CAD build for the part. Positions are in the model's coordinates, mm. Round coordinates to 2 decimals unless told otherwise and drop trailing zeros. Write each loop counter-clockwise with the first axis right and the second up, starting at its lowest first coordinate (ties: lowest second). Pieces come first, ordered by that corner, then holes. Notation, with made-up numbers: (13.5, -15.5) - (19.5, -15.5) arc R32 ccw to (19.5, 18.5) - close; hole circle Ø11 at (-31.5, 59). An arc over 180 degrees is marked (long way). Answer in a Markdown table with one row per item.
```python
from build123d import *

# Parameters (mm, degrees)
SKETCH_1_R      = 3.2
SKETCH_1_R_2    = 1.6
EXTRUDE_1_DEPTH = 3


with BuildPart() as part:
    # 草图1 → 凸台-拉伸1 (new body)
    with BuildSketch(Plane(origin=(0, 0, 0), x_dir=(1, 0, 0), z_dir=(0, 1, 0))):
        with BuildLine():
            Line((5, 0), (175, 0))
            ThreePointArc((175, 0), (178.535533906, 1.464466094), (180, 5))
            Line((180, 5), (180, 175))
            ThreePointArc((180, 175), (178.535533906, 178.535533906), (175, 180))
            Line((175, 180), (5, 180))
            ThreePointArc((5, 180), (1.464466094, 178.535533906), (0, 175))
            Line((0, 175), (0, 5))
            ThreePointArc((0, 5), (1.464466094, 1.464466094), (5, 0))
        make_face()
        with Locations(Location((8, 172, 0), (0, 0, 270))):
            Circle(SKETCH_1_R, mode=Mode.SUBTRACT)
        with Locations(Location((172, 172, 0), (0, 0, 270))):
            Circle(SKETCH_1_R, mode=Mode.SUBTRACT)
        with Locations(Location((8, 8, 0), (0, 0, 270))):
            Circle(SKETCH_1_R, mode=Mode.SUBTRACT)
        with Locations(Location((172, 8, 0), (0, 0, 270))):
            Circle(SKETCH_1_R, mode=Mode.SUBTRACT)
        with Locations(Location((74.5, 175, 0), (0, 0, 270))):
            Circle(SKETCH_1_R_2, mode=Mode.SUBTRACT)
        with Locations(Location((74.5, 144, 0), (0, 0, 270))):
            Circle(SKETCH_1_R_2, mode=Mode.SUBTRACT)
        with Locations(Location((105.5, 144, 0), (0, 0, 90))):
            Circle(SKETCH_1_R_2, mode=Mode.SUBTRACT)
        with Locations(Location((105.5, 175, 0), (0, 0, 90))):
            Circle(SKETCH_1_R_2, mode=Mode.SUBTRACT)
        with Locations(Location((133.6, 172, 0), (0, 0, 270))):
            Circle(SKETCH_1_R_2, mode=Mode.SUBTRACT)
        with Locations(Location((133.6, 158, 0), (0, 0, 270))):
            Circle(SKETCH_1_R_2, mode=Mode.SUBTRACT)
        with Locations(Location((154, 169.5, 0), (0, 0, 270))):
            Circle(SKETCH_1_R_2, mode=Mode.SUBTRACT)
        with Locations(Location((154, 155.5, 0), (0, 0, 270))):
            Circle(SKETCH_1_R_2, mode=Mode.SUBTRACT)
        with Locations(Location((130, 135, 0), (0, 0, 270))):
            Circle(SKETCH_1_R_2, mode=Mode.SUBTRACT)
        with Locations(Location((130, 45, 0), (0, 0, 270))):
            Circle(SKETCH_1_R_2, mode=Mode.SUBTRACT)
        with Locations(Location((45, 137, 0), (0, 0, 270))):
            Circle(SKETCH_1_R_2, mode=Mode.SUBTRACT)
        with Locations(Location((45, 45, 0), (0, 0, 270))):
            Circle(SKETCH_1_R_2, mode=Mode.SUBTRACT)
        with Locations(Location((45, 126, 0), (0, 0, 270))):
            Circle(SKETCH_1_R_2, mode=Mode.SUBTRACT)
        with Locations(Location((45, 60, 0), (0, 0, 270))):
            Circle(SKETCH_1_R_2, mode=Mode.SUBTRACT)
        with Locations(Location((62, 45, 0), (0, 0, 270))):
            Circle(SKETCH_1_R_2, mode=Mode.SUBTRACT)
        with Locations(Location((62, 5, 0), (0, 0, 270))):
            Circle(SKETCH_1_R_2, mode=Mode.SUBTRACT)
        with Locations(Location((118, 45, 0), (0, 0, 270))):
            Circle(SKETCH_1_R_2, mode=Mode.SUBTRACT)
        with Locations(Location((118, 5, 0), (0, 0, 270))):
            Circle(SKETCH_1_R_2, mode=Mode.SUBTRACT)
        with Locations(Location((90, 90, 0), (0, 0, 270))):
            Circle(SKETCH_1_R_2, mode=Mode.SUBTRACT)
        with Locations(Location((90, 60, 0), (0, 0, 270))):
            Circle(SKETCH_1_R_2, mode=Mode.SUBTRACT)
        with Locations(Location((105, 75, 0), (0, 0, 270))):
            Circle(SKETCH_1_R_2, mode=Mode.SUBTRACT)
        with Locations(Location((75, 75, 0), (0, 0, 270))):
            Circle(SKETCH_1_R_2, mode=Mode.SUBTRACT)
        with Locations(Location((46, 5, 0), (0, 0, 270))):
            Circle(SKETCH_1_R_2, mode=Mode.SUBTRACT)
        with Locations(Location((46, 35, 0), (0, 0, 270))):
            Circle(SKETCH_1_R_2, mode=Mode.SUBTRACT)
        with Locations(Location((134, 35, 0), (0, 0, 270))):
            Circle(SKETCH_1_R_2, mode=Mode.SUBTRACT)
        with Locations(Location((134, 5, 0), (0, 0, 270))):
            Circle(SKETCH_1_R_2, mode=Mode.SUBTRACT)
    extrude(amount=EXTRUDE_1_DEPTH)


solid = part.part
```
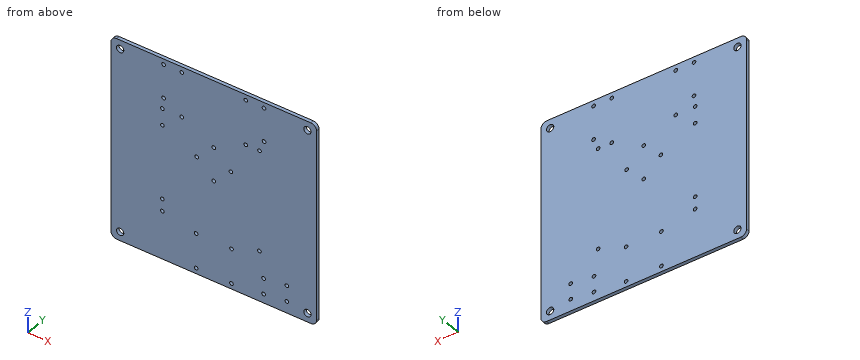
Q1. Saw through at A-A on x = 8. List the corners of the cut face in (y, z).
Computed:
| item | result |
|---|---|
| outline | (0, -180) - (3, -180) - (3, -175.2) - (0, -175.2) - close; (0, -168.8) - (3, -168.8) - (3, -11.2) - (0, -11.2) - close; (0, -4.8) - (3, -4.8) - (3, 0) - (0, 0) - close |
Q2. Drill centre lines: line 1 (Z direction, x = 90, y = 2); line 2 (X direction, y = 0.7, z = -135); line 3 (X direction, y = 1.65, z = -8). Where is each one in solid material? Low to high.
Computed:
| item | result |
|---|---|
| line 1 | z = -180 to -91.6, -88.4 to -61.6, -58.4 to 0 |
| line 2 | x = 0 to 128.4, 131.6 to 180 |
| line 3 | x = 0 to 4.8, 11.2 to 168.8, 175.2 to 180 |
Q3. Flat gauge pin, fed straight in: pin 1 (3 mm diameter, centred on x = 45, z = -60, fed in from +Y). Where does the tip first touch, or does it go through?
Computed:
| item | result |
|---|---|
| pin 1 | passes through |
